Input: part model. Units: mm. Frame: model coordinates. Face numbers are marked on the shaded views. A direction names the side the tool comes from. Coordinates: 2 decimals unless noted, no trailing zeros. Write each loop counter-clockwise with the first axis right and the second up, starting at its lowest first coordinate (ties: lowest second). Pieces come first, ordered by that corner, then holes. Notation, with made-up numbers: (38, -31) - (61, -31) arc R8 cw to (61, -19) - close; hole circle Ø11 at (44.5, 59.5). An arc over 180 degrees is marked (long way). Use a Markdown table: item, result. Add a question column.
Q1. Mould query, pull axis Y, two halves, no side actions, for the marked faces 5, 6 and 7. Classes: released by +Y, released by -Y, zero draft, split by the parting line, or undercut.
Q2. Section query A-A (x = 16.5). Return the cut outline in (y, z), then the cut area to 4 significant figures.
Q3. Set-up query: the marked faces 1, 2, 3 and 4. Return all of +Z, -Z, +X, -X, +Y, -Y with unobstructed straight access to the full face (end or side cutting, diameter ignored); none if empty.
Q4. Section query C-C (x = 25). Return the cut outline in (y, z).
Q5. Section query D-D (y = 3.75). Return the cut outline in (x, z), then the cut area to 3 significant figures.
Q6. Material intervals for probe 1 along Y at (x, z) = (31.5, 0.8); probe 2 along X at (y, z) = (14.75, 1.95); probe 3 along Z at (x, y) = (18, 4.25), sorted ascending. Write a range as from..to.
Q7. Section query B-B (y = 17). Return the cut outline in (x, z), then the cut area to 3 significant figures.
Q8. Pin query (flat end, axial travel): P1, Ø0.6, axis at x = 4, z = 2, coming from the +Y side; P2, Ø1.5, axis at x = 14.5, z = 3, coming from the +Y side; P3, Ø1, axis at y = 7, z = 2.5, coming from the +X side; P4, Ø2.5, axis at x = 24.5, y = 2.5, coming from the +Z side. Return the tip coordinate at first contact, or that it passes through.
from build123d import *

# Parameters (mm, degrees)
SKETCH_1_W          = 33
SKETCH_1_H          = 23
EXTRUDE_1_DEPTH     = 1.5
SKETCH_2_W          = 12
SKETCH_2_H          = 1.5
CUT_EXTRUDE_1_DEPTH = 41.252329125
SKETCH_3_R          = 0.75
CUT_EXTRUDE_2_DEPTH = 41.252329125
SKETCH_4_W          = 4
SKETCH_4_H          = 2
EXTRUDE_2_DEPTH     = 2
SKETCH_5_W          = 3
SKETCH_5_H          = 5
EXTRUDE_3_DEPTH     = 2
SKETCH_6_W          = 6.5
SKETCH_6_H          = 6.5
EXTRUDE_4_DEPTH     = 3
SKETCH_7_W          = 7
SKETCH_7_H          = 5
EXTRUDE_5_DEPTH     = 2.5


with BuildPart() as part:
    # 草图1 → 凸台-拉伸1 (new body)
    with BuildSketch(Plane.XY):
        with Locations((16.5, 11.5)):
            Rectangle(SKETCH_1_W, SKETCH_1_H)
    extrude(amount=EXTRUDE_1_DEPTH)

    # 草图2 → 切除-拉伸1 (cut, through all)
    with BuildSketch(Plane.XY.offset(1.5)):
        with Locations((24, 0.75)):
            Rectangle(SKETCH_2_W, SKETCH_2_H)
    extrude(amount=-CUT_EXTRUDE_1_DEPTH, mode=Mode.SUBTRACT)

    # 草图3 → 切除-拉伸2 (cut, through all)
    with BuildSketch(Plane.XY.offset(1.5)):
        with Locations((31.5, 1.2)):
            Circle(SKETCH_3_R)
        with Locations((16.5, 1.2)):
            Circle(SKETCH_3_R)
    extrude(amount=-CUT_EXTRUDE_2_DEPTH, mode=Mode.SUBTRACT)

    # 草图4 → 凸台-拉伸2 (add)
    with BuildSketch(Plane.XY.offset(1.5)):
        with Locations((4, 7)):
            Rectangle(SKETCH_4_W, SKETCH_4_H)
    extrude(amount=EXTRUDE_2_DEPTH)

    # 草图5 → 凸台-拉伸3 (add)
    with BuildSketch(Plane.XY.offset(1.5)):
        with Locations((27.5, 15.5)):
            Rectangle(SKETCH_5_W, SKETCH_5_H)
    extrude(amount=EXTRUDE_3_DEPTH)

    # 草图6 → 凸台-拉伸4 (add)
    with BuildSketch(Plane.XY.offset(1.5)):
        with Locations((3.35, 15.75)):
            Rectangle(SKETCH_6_W, SKETCH_6_H)
    extrude(amount=EXTRUDE_4_DEPTH)

    # 草图7 → 凸台-拉伸5 (add)
    with BuildSketch(Plane.XY.offset(1.5)):
        with Locations((24.039083368, 3)):
            Rectangle(SKETCH_7_W, SKETCH_7_H)
    extrude(amount=EXTRUDE_5_DEPTH)


solid = part.part
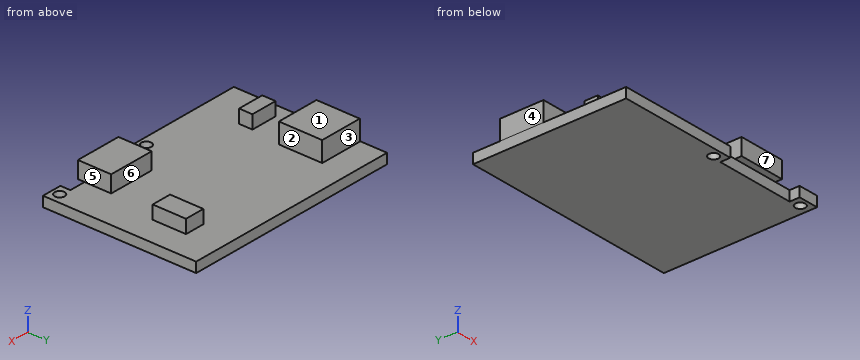
Values follow:
| question | item | result |
|---|---|---|
| 1 | face 5 | zero draft |
| 1 | face 6 | undercut |
| 1 | face 7 | released by -Y |
| 2 | outline | (0, 0) - (0.45, 0) - (0.45, 1.5) - (0, 1.5) - close; (1.95, 0) - (23, 0) - (23, 1.5) - (1.95, 1.5) - close |
| 2 | area | 32.25 mm2 |
| 3 | face 1 | +Z, +X, -X, +Y, -Y |
| 3 | face 2 | +Z, +Y, -Y |
| 3 | face 3 | +Z, +X, -X, +Y |
| 3 | face 4 | +Z, -X, +Y, -Y |
| 4 | outline | (0.5, 1.5) - (1.5, 1.5) - (1.5, 0) - (23, 0) - (23, 1.5) - (5.5, 1.5) - (5.5, 4) - (0.5, 4) - close |
| 5 | outline | (0, 0) - (33, 0) - (33, 1.5) - (27.54, 1.5) - (27.54, 4) - (20.54, 4) - (20.54, 1.5) - (0, 1.5) - close |
| 5 | area | 67.0 mm2 |
| 6 | probe 1 | 0..0.45, 1.95..23 |
| 6 | probe 2 | 0.1..6.6, 26..29 |
| 6 | probe 3 | 0..1.5 |
| 7 | outline | (0, 0) - (33, 0) - (33, 1.5) - (29, 1.5) - (29, 3.5) - (26, 3.5) - (26, 1.5) - (6.6, 1.5) - (6.6, 4.5) - (0.1, 4.5) - (0.1, 1.5) - (0, 1.5) - close |
| 7 | area | 75.0 mm2 |
| 8 | P1 | y = 19 |
| 8 | P2 | through |
| 8 | P3 | x = 6 |
| 8 | P4 | z = 4 |
